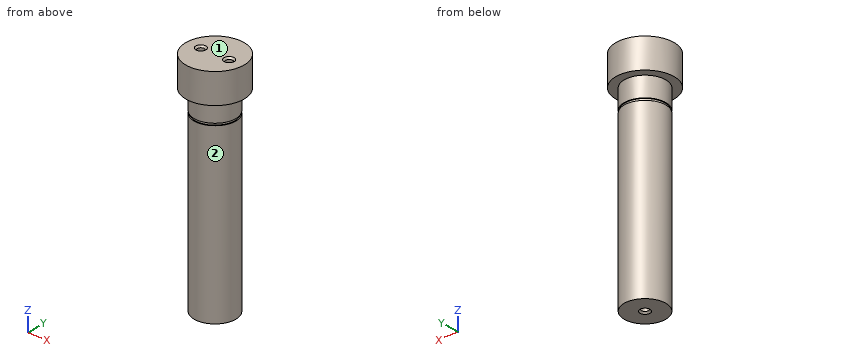
Solid Edge part; units mm, degrees
sketch "Sketch1" plane through (0, 0, 0) normal (0, -1, 0) x (1, 0, 0)
  line L0 (0, 0) -> (0, 136)
  line L1 (0, 136) -> (17.5, 136)
  line L2 (17.5, 136) -> (17.5, 118)
  line L3 (17.5, 118) -> (12.5, 118)
  line L4 (12.5, 118) -> (12.5, 106)
  line L5 (12.5, 106) -> (11.95, 106)
  line L6 (11.95, 106) -> (11.95, 104.7)
  line L7 (11.95, 104.7) -> (12.5, 104.7)
  line L8 (12.5, 104.7) -> (12.5, 0)
  line L9 (12.5, 0) -> (0, 0)
revolve "RevolvedProtrusion1" add sketch "Sketch1" angle 360 about axis through (0, 0, 0) along (0, 0, 1)
hole "Hole1" at (8.75, 0, 136) direction (0, 0, -1) diameter 4.134 depth 15 start chamfer 1 start chamfer angle 45
hole "Hole2" at (-8.75, 0, 136) direction (0, 0, -1) diameter 4.134 depth 15 start chamfer 1 start chamfer angle 45
hole "v_1" at (0, 0, 0) direction (0, 0, 1) diameter 4.134 depth 15 start chamfer 1 start chamfer angle 45
Check sheet for the modelled part. Datum: model origin and axes. Units: mm. Face numbers are marked on the shaded views. A direction names the side the tool comes from. Round coordinates to 2 decimals unless told otherwise and drop trailing zeros. Write each loop counter-clockwise with the first axis right and the second up, starting at its lowest first coordinate (ties: lowest second). Pieces come first, ordered by that corner, then holes. Notation, with made-up numbers: (-31, -40) -> (8, -40) arc R17 cw to (8, -30) -> close; hole circle Ø4 at (83.25, -21.75). An arc over 180 degrees is marked (long way). One line per question, with ' | ' between items. Start each with the question number.
1. Scan lines: line 1 along Y through (x, z) = (0, 10); line 2 along Z through (x, y) = (11.5, -4); line 3 along Z through (x, y) = (-8, 15). Record each from-to range of solid material in increasing order. Write a range as from..to.
2. Depth check by flat-ended pin: pin 1 (2 mm diameter, centred on y = -8, z = 89.5, fed in from +X); pin 2 (12 mm diameter, centred on y = 10.5, z = 59.5, fed in from -X); pin 3 (2 mm diameter, centred on x = -12.5, z = 44, fed in from -Y); pin 4 (3 mm diameter, centred on x = 12, y = -1.5, fed in from -Z). Enter the tip coordinate at first touch or a pass-through.
3. Sectioned sample at C-C, the plane x = 0. Record the cut outline in (y, z).
4. Sectioned sample at B-B, the plane z = 13.5. Record the cut outline in (x, y), then the cut area to 3 significant figures.
5. Sectioned sample at D-D, the plane z = 42.5. Record the cut outline in (x, y).
6. Set-up check for the marked faces 1 and 2: record each of +Z, -Z, +X, -X, +Y, -Y from which the full face is reachable in a straight line by a thin tool's end or side.
Taken from the geometry:
1) line 1: y = -12.5..-2.07, 2.07..12.5 | line 2: z = 0..104.7, 106..136 | line 3: z = 118..136
2) pin 1: stops at x = 10.36 | pin 2: stops at x = -11.66 | pin 3: stops at y = -4.9 | pin 4: stops at z = 0
3) outline: (-17.5, 118) -> (-12.5, 118) -> (-12.5, 106) -> (-11.95, 106) -> (-11.95, 104.7) -> (-12.5, 104.7) -> (-12.5, 0) -> (-3.07, 0) -> (-2.07, 1) -> (-2.07, 15) -> (2.07, 15) -> (2.07, 1) -> (3.07, 0) -> (12.5, 0) -> (12.5, 104.7) -> (11.95, 104.7) -> (11.95, 106) -> (12.5, 106) -> (12.5, 118) -> (17.5, 118) -> (17.5, 136) -> (-17.5, 136) -> close
4) outline: circle Ø25 at (0, 0); hole circle Ø4.13 at (0, 0) | area: 477 mm^2
5) outline: circle Ø25 at (0, 0)
6) face 1: +Z, +X, -X, +Y, -Y | face 2: -Z
